Can you work these out from the model? Positions are in its coordinate system, mm. A direction names the side the tool comes from. Give positions to 0.01 mm unless a question says otherwise; leave off trailing zeros. Loops run counter-clockwise (first coordinate to the right, second up) from the corner with the lowest first, then second, coordinate; pieces in that order, holes last. Notation, with made-up numbers: (-9.75, 2.5) - (10.25, 2.5) arc R14 cw to (10.25, 21.5) - close; hole circle Ø5 at (-25, 57.25). An arc over 180 degrees is marked (long way). Answer in a Markdown table with one row per item.
from build123d import *

# Parameters (mm, degrees)
SKETCH1_W             = 130
SKETCH1_H             = 80
BOSS_EXTRUDE1_DEPTH   = 10
FILLET1_R             = 4
F_4_0MM_DOWEL_HOLE1_D = 4
MIRROR2_COPY_1_D      = 4
SKETCH8_W             = 95
SKETCH8_H             = 55
CUT_EXTRUDE4_DEPTH    = 10
SKETCH4_W             = 106.5
SKETCH4_H             = 68
CUT_EXTRUDE1_DEPTH    = 5.1
SKETCH6_W             = 7
SKETCH6_H             = 64
CUT_EXTRUDE3_DEPTH    = 10
FILLET3_R             = 4
SKETCH10_W            = 66.25
SKETCH10_H            = 2.5
CUT_EXTRUDE6_DEPTH    = 10
SKETCH12_W            = 5.983903777
SKETCH12_H            = 17.5
SKETCH12_W_2          = 5.75
SKETCH12_H_2          = 39
CUT_EXTRUDE7_DEPTH    = 10
SKETCH13_W            = 86.5
SKETCH13_H            = 6.5
CUT_EXTRUDE8_DEPTH    = 10
SKETCH14_W            = 5.75
SKETCH14_H            = 39
CUT_EXTRUDE9_DEPTH    = 10
SKETCH15_W            = 5.75
SKETCH15_H            = 17.5
CUT_EXTRUDE10_DEPTH   = 10
SKETCH16_W            = 94.766096223
SKETCH16_H            = 6.5
CUT_EXTRUDE11_DEPTH   = 10
FILLET4_R             = 2


with BuildPart() as part:
    # Sketch1 → Boss-Extrude1 (new body)
    with BuildSketch(Plane.XY):
        Rectangle(SKETCH1_W, SKETCH1_H)
    extrude(amount=BOSS_EXTRUDE1_DEPTH)

    # Fillet1
    fillet1_edges = [part.edges().sort_by_distance(p)[0] for p in [
        (65, -40, 5),
        (-65, -40, 5),
        (-65, 40, 5),
        (65, 40, 5),
    ]]
    fillet(fillet1_edges, radius=FILLET1_R)

    # Ø4.0mm Dowel Hole1 (through all)
    with Locations(Plane.XY.offset(10)):
        with Locations((-61, 36)):
            f_4_0mm_dowel_hole1 = Hole(F_4_0MM_DOWEL_HOLE1_D / 2)

    # Mirror1: Ø4.0mm Dowel Hole1 across plane
    add(f_4_0mm_dowel_hole1.mirror(Plane(origin=(0, 0, 0), x_dir=(0, 0, 1), z_dir=(1, 0, 0))), mode=Mode.SUBTRACT)

    # Mirror2: Ø4.0mm Dowel Hole1 across plane
    add(f_4_0mm_dowel_hole1.mirror(Plane.ZX), mode=Mode.SUBTRACT)

    # Mirror2 copy 1 (through all)
    with Locations(Plane(origin=(0, 0, 10), x_dir=(-1, 0, 0), z_dir=(0, 0, 1))):
        with Locations((-61, 36)):
            Hole(MIRROR2_COPY_1_D / 2)

    # Sketch8 → Cut-Extrude4 (cut)
    with BuildSketch(Plane.XY.offset(10)):
        Rectangle(SKETCH8_W, SKETCH8_H)
    extrude(amount=-CUT_EXTRUDE4_DEPTH, mode=Mode.SUBTRACT)

    # Sketch4 → Cut-Extrude1 (cut)
    with BuildSketch(Plane.XY.offset(10)):
        Rectangle(SKETCH4_W, SKETCH4_H)
    extrude(amount=-CUT_EXTRUDE1_DEPTH, mode=Mode.SUBTRACT)

    # Sketch6 → Cut-Extrude3 (cut)
    with BuildSketch(Plane.XY.offset(10)):
        with Locations((61.5, 0)):
            Rectangle(SKETCH6_W, SKETCH6_H)
    cut_extrude3 = extrude(amount=-CUT_EXTRUDE3_DEPTH, mode=Mode.SUBTRACT)

    # Mirror6: Cut-Extrude3 across plane
    add(cut_extrude3.mirror(Plane(origin=(0, 0, 0), x_dir=(0, 0, 1), z_dir=(1, 0, 0))), mode=Mode.SUBTRACT)

    # Fillet3
    fillet3_edges = [part.edges().sort_by_distance(p)[0] for p in [
        (65, -32, 5),
        (65, 32, 5),
        (-65, -32, 5),
        (-65, 32, 5),
    ]]
    fillet(fillet3_edges, radius=FILLET3_R - 0.0001)  # a hair under: the kernel refuses the full size

    # Sketch10 → Cut-Extrude6 (cut)
    with BuildSketch(Plane.XY.offset(10)):
        with Locations((-18.125, -35.25)):
            Rectangle(SKETCH10_W, SKETCH10_H)
    extrude(amount=-CUT_EXTRUDE6_DEPTH, mode=Mode.SUBTRACT)

    # Sketch12 → Cut-Extrude7 (cut)
    with BuildSketch(Plane.XY.offset(4.9)):
        with Locations((-50.258048112, -25.25)):
            Rectangle(SKETCH12_W, SKETCH12_H)
        with Locations((-50.375, 8)):
            Rectangle(SKETCH12_W_2, SKETCH12_H_2)
    extrude(amount=-CUT_EXTRUDE7_DEPTH, mode=Mode.SUBTRACT)

    # Sketch13 → Cut-Extrude8 (cut)
    with BuildSketch(Plane.XY.offset(4.9)):
        with Locations((0, 30.75)):
            Rectangle(SKETCH13_W, SKETCH13_H)
    extrude(amount=-CUT_EXTRUDE8_DEPTH, mode=Mode.SUBTRACT)

    # Sketch14 → Cut-Extrude9 (cut)
    with BuildSketch(Plane.XY.offset(4.9)):
        with Locations((50.375, 8)):
            Rectangle(SKETCH14_W, SKETCH14_H)
    extrude(amount=-CUT_EXTRUDE9_DEPTH, mode=Mode.SUBTRACT)

    # Sketch15 → Cut-Extrude10 (cut)
    with BuildSketch(Plane.XY.offset(4.9)):
        with Locations((50.375, -25.25)):
            Rectangle(SKETCH15_W, SKETCH15_H)
    extrude(amount=-CUT_EXTRUDE10_DEPTH, mode=Mode.SUBTRACT)

    # Sketch16 → Cut-Extrude11 (cut)
    with BuildSketch(Plane.XY.offset(4.9)):
        with Locations((0.116951888, -30.75)):
            Rectangle(SKETCH16_W, SKETCH16_H)
    extrude(amount=-CUT_EXTRUDE11_DEPTH, mode=Mode.SUBTRACT)

    # Fillet4
    fillet4_edges = [part.edges().sort_by_distance(p)[0] for p in [
        (-47.5, -16.5, 2.45),
        (-47.5, -11.5, 2.45),
        (43.25, 27.5, 2.45),
        (-43.25, 27.5, 2.45),
        (47.5, -11.5, 2.45),
        (47.5, -16.5, 2.45),
    ]]
    fillet(fillet4_edges, radius=FILLET4_R)


solid = part.part
Q1. If we mould it in two halves opening along X, with no side actions, what happens to faces 6 (the face through (-58, 0, 5)), 7 (the face through (43.25, 32, 2)), 8 (the face through (63.859, 38.797, 5.07))? For each: released by +X, released by -X, zero draft, split by the parting line, or undercut.
Checked values:
| item | result |
|---|---|
| face 6 | released by -X |
| face 7 | undercut |
| face 8 | released by +X |
Q2. Imagine slicing it at C-C, the plane z = 2.25. Count the separate pieces of the cut face and the enclosed holes in it, and give its area (3 significant figures).
Checked values:
| item | result |
|---|---|
| separate pieces | 1 |
| enclosed holes | 5 |
| area | 2,200 mm² |
Q3. Imagine slicing it at B-B, the plane x = -6. Write out the boundary of the cut face in (y, z), and give its area (3 significant figures).
Checked values:
| item | result |
|---|---|
| outline | (-40, 0) - (-36.5, 0) - (-36.5, 10) - (-40, 10) - close; (34, 0) - (40, 0) - (40, 10) - (34, 10) - close |
| area | 95.0 mm² |
Q4. For pin 1 (5 mm diameter, centred on y = -6, z = 4.5, fed in from -X); pin 2 (3 mm diameter, centred on x = 48, y = 30.5, fed in from +Z); pin 3 (6 mm diameter, centred on y = -12, z = 6, fed in from +X), each with a flat end and sliding along its axis, tell me the tip position at first contact or that it passes through.
Checked values:
| item | result |
|---|---|
| pin 1 | stops at x = -58 |
| pin 2 | stops at z = 4.9 |
| pin 3 | stops at x = 58 |
Q5. On a 3-axis mill with a long thin cutter (end or side, diameter ignored), from which of +Z, -Z, +X, -X, +Y, -Y can I reach the whole of each face in a straight line? I mean faces 1 (the face through (63.859, 33.203, 4.93)), 2 (the face through (-51, -11.5, 2)), 3 (the face through (-63.859, -33.203, 4.93)), 4 (the face through (5, 36, 0)), 5 (the face through (48, 31, 4.9)). Say none if no direction works.
Checked values:
| item | result |
|---|---|
| face 1 | +Z, -Z, +X |
| face 2 | +Z, -Z |
| face 3 | +Z, -Z, -X |
| face 4 | -Z, +X, -X, +Y, -Y |
| face 5 | +Z |
Q6. If I drill on line 1 (Y direction, x = -53, z = 4.25); line 2 (Y direction, x = -61, z = 6); line 3 (X direction, y = 19.5, z = 5), over which ranges is the centre line in solid material (lowest first)? Write a range as [from, to].
Checked values:
| item | result |
|---|---|
| line 1 | y = [-40, -34], [-16.5, -11.5], [27.5, 40] |
| line 2 | y = [-40, -38], [-34, -32], [32, 34], [38, 40] |
| line 3 | x = [-58, -53.25], [53.25, 58] |
Q7. Imagine slicing it at A-A, the plane y = -23.5. Write out the boundary of the cut face in (x, z), and give its area (3 significant figures).
Checked values:
| item | result |
|---|---|
| outline | (-58, 0) - (-53.25, 0) - (-53.25, 10) - (-58, 10) - close; (53.25, 0) - (58, 0) - (58, 10) - (53.25, 10) - close |
| area | 95.0 mm² |
